Geometry check sheet. Reference: the model listing, model coordinates, mm. A direction names the side the tool comes from. Round coordinates to 2 decimals unless told otherwise and drop trailing zeros. Write each loop counter-clockwise with the first axis right and the second up, starting at its lowest first coordinate (ties: lowest second). Pieces come first, ordered by that corner, then holes. Notation, with made-up numbers: (76, 7.5) - (106, 7.5) arc R21 ccw to (106, 38.5) - close; hole circle Ø7 at (67.25, -39.75). An arc over 180 degrees is marked (long way). Return JSON: item names as keys, results as strings. Group by question number.
from build123d import *

# Parameters (mm, degrees)
BOSS_EXTRUDE1_DEPTH     = 22.7
SKETCH5_R               = 1.5
CUT_EXTRUDE1_DEPTH      = 70
SKETCH6_R               = 11.25
CUT_EXTRUDE3_DEPTH      = 17.25
CUT_EXTRUDE3_DEPTH_BACK = 17.25
SKETCH7_R               = 2
CUT_EXTRUDE4_DEPTH      = 3
SKETCH8_W               = 6.5
SKETCH8_H               = 75.6
CUT_EXTRUDE5_DEPTH      = 58
CUT_EXTRUDE5_DEPTH_BACK = 66
SKETCH9_R               = 2.35
SKETCH9_R_2             = 1.55
CUT_EXTRUDE7_DEPTH      = 4
SKETCH9_3_R             = 1.55
CUT_EXTRUDE20_DEPTH     = 12
SKETCH21_R              = 2.35
SKETCH21_R_2            = 1.55
CUT_EXTRUDE22_DEPTH     = 4
SKETCH21_2_R            = 1.55
CUT_EXTRUDE23_DEPTH     = 12
SKETCH19_R              = 2.35
SKETCH19_R_2            = 1.55
CUT_EXTRUDE24_DEPTH     = 4
SKETCH19_2_R            = 1.55
CUT_EXTRUDE25_DEPTH     = 12
SKETCH20_R              = 2.35
SKETCH20_R_2            = 1.55
CUT_EXTRUDE26_DEPTH     = 4
SKETCH20_2_R            = 1.55
CUT_EXTRUDE27_DEPTH     = 12
FILLET2_R               = 2.5
BOSS_EXTRUDE2_DEPTH     = 0.5


with BuildPart() as part:
    # Sketch4 → Boss-Extrude1 (new body)
    with BuildSketch(Plane.XY):
        with BuildLine():
            Line((-5, 37.8), (-5, 12))
            ThreePointArc((-5, 12), (-9.192388155, 9.192388155), (-12, 5))
            Line((-12, 5), (-37.8, 5))
            Line((-37.8, 5), (-37.8, -5))
            Line((-37.8, -5), (-12, -5))
            ThreePointArc((-12, -5), (-9.192388155, -9.192388155), (-5, -12))
            Line((-5, -12), (-5, -37.8))
            Line((-5, -37.8), (5, -37.8))
            Line((5, -37.8), (5, -12))
            ThreePointArc((5, -12), (9.192388155, -9.192388155), (12, -5))
            Line((12, -5), (37.8, -5))
            Line((37.8, -5), (37.8, 5))
            Line((37.8, 5), (12, 5))
            ThreePointArc((12, 5), (9.192388155, 9.192388155), (5, 12))
            Line((5, 12), (5, 37.8))
            Line((5, 37.8), (-5, 37.8))
        make_face()
    extrude(amount=-BOSS_EXTRUDE1_DEPTH)

    # Sketch5 → Cut-Extrude1 (cut)
    with BuildSketch(Plane.XY):
        with Locations((2.184887392, 8.154110756)):
            Circle(SKETCH5_R)
        with Locations((-8.154110756, -2.184887392)):
            Circle(SKETCH5_R)
        with Locations((5.969223364, -5.969223364)):
            Circle(SKETCH5_R)
        with BuildLine():
            Line((-5, 16.456455054), (-3.523070126, 11.621395871))
            ThreePointArc((-3.523070126, 11.621395871), (-4.596194078, 4.596194078), (-11.621395871, 3.523070126))
            Line((-11.621395871, 3.523070126), (-16.456455054, 5))
            Line((-16.456455054, 5), (-14.526937175, 6.929517879))
            ThreePointArc((-14.526937175, 6.929517879), (-13.081475452, 13.081475452), (-6.929517879, 14.526937175))
            Line((-6.929517879, 14.526937175), (-5, 16.456455054))
        make_face()
    extrude(amount=-CUT_EXTRUDE1_DEPTH, mode=Mode.SUBTRACT)

    # Sketch6 → Cut-Extrude3 (cut, two sides)
    with BuildSketch(Plane(origin=(0, 0, -22.7), x_dir=(-1, 0, 0), z_dir=(0, 0, -1))) as cut_extrude3_sk:
        Circle(SKETCH6_R)
    extrude(amount=CUT_EXTRUDE3_DEPTH, mode=Mode.SUBTRACT)
    extrude(cut_extrude3_sk.sketch, amount=-CUT_EXTRUDE3_DEPTH_BACK, mode=Mode.SUBTRACT)

    # Sketch7 → Cut-Extrude4 (cut)
    with BuildSketch(Plane(origin=(0, 0, -5.45), x_dir=(-1, 0, 0), z_dir=(0, 0, -1))):
        with Locations((-2.184887392, 8.154110756)):
            Circle(SKETCH7_R)
        with Locations((-5.969223364, -5.969223364)):
            Circle(SKETCH7_R)
        with Locations((8.154110756, -2.184887392)):
            Circle(SKETCH7_R)
    extrude(amount=-CUT_EXTRUDE4_DEPTH, mode=Mode.SUBTRACT)

    # Sketch8 → Cut-Extrude5 (cut, two sides)
    with BuildSketch(Plane.ZY.offset(5)) as cut_extrude5_sk:
        with Locations((-19.45, 0)):
            Rectangle(SKETCH8_W, SKETCH8_H)
    extrude(amount=CUT_EXTRUDE5_DEPTH, mode=Mode.SUBTRACT)
    extrude(cut_extrude5_sk.sketch, amount=-CUT_EXTRUDE5_DEPTH_BACK, mode=Mode.SUBTRACT)

    # Sketch9 → Cut-Extrude7 (cut)
    with BuildSketch(Plane(origin=(0, 37.8, 0), x_dir=(1, 0, 0), z_dir=(0, 1, 0))):
        with Locations((0, 5)):
            Circle(SKETCH9_R)
        with Locations((0, 5)):
            Circle(SKETCH9_R_2, mode=Mode.SUBTRACT)
    extrude(amount=-CUT_EXTRUDE7_DEPTH, mode=Mode.SUBTRACT)

    # Sketch9_3 → Cut-Extrude20 (cut)
    with BuildSketch(Plane(origin=(0, 37.8, 0), x_dir=(1, 0, 0), z_dir=(0, 1, 0))):
        with Locations((0, 5)):
            Circle(SKETCH9_3_R)
    extrude(amount=-CUT_EXTRUDE20_DEPTH, mode=Mode.SUBTRACT)

    # Sketch21 → Cut-Extrude22 (cut)
    with BuildSketch(Plane.ZY.offset(37.8)):
        with Locations((-5, 0)):
            Circle(SKETCH21_R)
        with Locations((-5, 0)):
            Circle(SKETCH21_R_2, mode=Mode.SUBTRACT)
    extrude(amount=-CUT_EXTRUDE22_DEPTH, mode=Mode.SUBTRACT)

    # Sketch21_2 → Cut-Extrude23 (cut)
    with BuildSketch(Plane.ZY.offset(37.8)):
        with Locations((-5, 0)):
            Circle(SKETCH21_2_R)
    extrude(amount=-CUT_EXTRUDE23_DEPTH, mode=Mode.SUBTRACT)

    # Sketch19 → Cut-Extrude24 (cut)
    with BuildSketch(Plane(origin=(37.8, 0, 0), x_dir=(0, 0, -1), z_dir=(1, 0, 0))):
        with Locations((5, 0)):
            Circle(SKETCH19_R)
        with Locations((5, 0)):
            Circle(SKETCH19_R_2, mode=Mode.SUBTRACT)
    extrude(amount=-CUT_EXTRUDE24_DEPTH, mode=Mode.SUBTRACT)

    # Sketch19_2 → Cut-Extrude25 (cut)
    with BuildSketch(Plane(origin=(37.8, 0, 0), x_dir=(0, 0, -1), z_dir=(1, 0, 0))):
        with Locations((5, 0)):
            Circle(SKETCH19_2_R)
    extrude(amount=-CUT_EXTRUDE25_DEPTH, mode=Mode.SUBTRACT)

    # Sketch20 → Cut-Extrude26 (cut)
    with BuildSketch(Plane.XZ.offset(37.8)):
        with Locations((0, -5)):
            Circle(SKETCH20_R)
        with Locations((0, -5)):
            Circle(SKETCH20_R_2, mode=Mode.SUBTRACT)
    extrude(amount=-CUT_EXTRUDE26_DEPTH, mode=Mode.SUBTRACT)

    # Sketch20_2 → Cut-Extrude27 (cut)
    with BuildSketch(Plane.XZ.offset(37.8)):
        with Locations((0, -5)):
            Circle(SKETCH20_2_R)
    extrude(amount=-CUT_EXTRUDE27_DEPTH, mode=Mode.SUBTRACT)

    # Fillet2
    fillet2_edges = [part.edges().sort_by_distance(p)[0] for p in [
        (-4.596194078, 4.596194078, 0),
    ]]
    fillet(fillet2_edges, radius=FILLET2_R)

    # Sketch22 → Boss-Extrude2 (add)
    with BuildSketch(Plane(origin=(0, 0, -5.45), x_dir=(-1, 0, 0), z_dir=(0, 0, -1))):
        Polygon((1.099038462, 3.175), (0.814102564, 3.175), (0.814102564, 1.872435897), (-0.814102564, 1.872435897), (-0.814102564, 3.175), (-1.099038462, 3.175), (-1.099038462, 0), (-0.814102564, 0), (-0.814102564, 1.546794872), (0.814102564, 1.546794872), (0.814102564, 0), (1.099038462, 0), align=None)
    extrude(amount=BOSS_EXTRUDE2_DEPTH)


solid = part.part
1. Section check A-A (x = -32). Enter the section's corners in (y, z), and give its area (3 significant figures).
2. Depth check by flat-ended pin: pin 1 Ø6 at (x, z) = (-16.5, -6) entering from +Y; pin 2 Ø0.6 at (y, z) = (1, -5.5) entering from +X; pin 3 Ø2 at (x, z) = (16.5, -13.5) entering from -Y. Enter the tip coordinate at first touch or a pass-through.
3. Tool access check on faces 4 (the face through (-6.156, -2.097, -3.971)), 5 (the face through (-4.27, 14.07, -7.99)), 6 (the face through (-29.86, 0.07, -6.55)). Record the directions out of +Z, -Z, +X, -X, +Y, -Y that give a thin tool (end or side, any length) a straight path to the whole face; none if there is none.
4. Section check B-B (y = 21). Enter the section's corners in (x, z).
5. Section check C-C (z = -14.25). Enter the section's corners in (x, y), and give its area (3 significant figures).
6. Mould release check, pull along X, two halves, no side actions. Record for faces 1 (the face through (-5, -25, -8)), 2 (the face through (0.715, -29.856, -6.375)), 3 (the face through (25, -5, -8)): pulls with the +X half, pulls with the -X half, needs draft (parallel to the pull), parting line crosses it, or undercut.
7. Material ranges on line 1 along Y through (x, z) = (35.4, -5); line 2 along X through (y, z) = (-0.5, -13.25); line 3 along Z through (x, y) = (0, -30), recorded low to high.
Result sheet:
{
 "1": {"outline": "(-5, -16.2) - (5, -16.2) - (5, 0) - (-5, 0) - close; hole circle Ø3.1 at (0, -5)", "area": "154 mm²"},
 "2": {"pin 1": "stops at y = 5", "pin 2": "stops at x = 25.8", "pin 3": "stops at y = -5"},
 "3": {"face 4": "-Z", "face 5": "+Z, -Z, -X", "face 6": "-X"},
 "4": {"outline": "(-5, -16.2) - (5, -16.2) - (5, 0) - (-5, 0) - close"},
 "5": {"outline": "(-37.8, -5) - (-12, -5) arc R13 ccw to (-5, -12) - (-5, -37.8) - (5, -37.8) - (5, -12) arc R13 ccw to (12, -5) - (37.8, -5) - (37.8, 5) - (12, 5) arc R13 ccw to (5, 12) - (5, 37.8) - (-5, 37.8) - (-5, 16.46) - (-3.52, 11.62) arc R6 cw to (-3.17, 10.8) arc R11.25 cw (long way) to (-10.8, 3.17) arc R6 cw to (-11.62, 3.52) - (-16.46, 5) - (-37.8, 5) - close", "area": "1,110 mm²"},
 "6": {"face 1": "pulls with the -X half", "face 2": "undercut", "face 3": "needs draft"},
 "7": {"line 1": "y = -5 to -2.35, 2.35 to 5", "line 2": "x = -37.8 to -11.24, 11.24 to 37.8", "line 3": "z = -16.2 to -6.55, -3.45 to 0"}
}
